```python
from build123d import *

# Parameters (mm, degrees)
SKETCH1_R               = 20.5
BOSS_EXTRUDE1_DEPTH     = 108
FILLET1_R               = 1
CUT_EXTRUDE1_REACH      = 130.166
CUT_EXTRUDE1_END_RADIUS = 18.5
CIRPATTERN1_COUNT       = 4
SKETCH7_R               = 0.75
BOSS_EXTRUDE2_DEPTH     = 0.5


# Read off the part's stored shape, not the designer's step: Shell1
with BuildPart() as part:
    # Sketch1 → Boss-Extrude1 (new body)
    with BuildSketch(Plane(origin=(0, 0, 0), x_dir=(1, 0, 0), z_dir=(0, 1, 0))):
        with Locations(Location((0, 0, 0), (0, 0, 270))):
            Circle(SKETCH1_R)
    extrude(amount=BOSS_EXTRUDE1_DEPTH)

    # Sketch3 → Revolve1 (revolve)
    with BuildSketch(Plane(origin=(0, 0, 0), x_dir=(0, 0, -1), z_dir=(1, 0, 0))):
        with BuildLine():
            Line((0, 116), (2.5, 116))
            Line((2.5, 116), (2.5, 114))
            ThreePointArc((2.5, 114), (5.663213274, 112.255038446), (8, 109.5))
            Line((8, 109.5), (8, 108))
            Line((8, 108), (0, 108))
            Line((0, 108), (0, 116))
        make_face()
    revolve(axis=Axis((0, 108, 0), (0, 1, 0)))

    # Fillet1
    fillet1_edges = [part.edges().sort_by_distance(p)[0] for p in [
        (0, 108, -20.5),
    ]]
    fillet(fillet1_edges, radius=FILLET1_R)

    # Shell1 outline → Shell1 (revolve, cut)
    with BuildSketch(Plane.XY):
        with BuildLine():
            Line((18.5, 0), (18.5, 106))
            Line((18.5, 106), (6, 106))
            Line((6, 106), (6, 108.933863711))
            ThreePointArc((6, 108.933863711), (3.622087212, 111.267143588), (0.5, 112.429570209))
            Line((0.5, 112.429570209), (0.5, 114))
            Line((0.5, 114), (0, 114))
            Line((0, 114), (0, 0))
            Line((0, 0), (18.5, 0))
        make_face()
    revolve(axis=Axis((0, 0, 0), (0, 1, 0)), mode=Mode.SUBTRACT)

    # Cut-Extrude1: up to this cylinder (the profile starts outside it)
    cut_extrude1_end = Plane(origin=(0, 80, 0), z_dir=(0, -1, 0)) * Cylinder(CUT_EXTRUDE1_END_RADIUS, 298.332, mode=Mode.PRIVATE)
    # Sketch4 → Cut-Extrude1 (cut, up to the surface)
    with BuildSketch(Plane(origin=(30, 0, 0), x_dir=(0, 0, -1), z_dir=(1, 0, 0)), mode=Mode.PRIVATE) as cut_extrude1_sk1:
        with BuildLine():
            Line((-7.5, 83), (7.5, 83))
            ThreePointArc((7.5, 83), (10.5, 80), (7.5, 77))
            Line((7.5, 77), (-7.5, 77))
            ThreePointArc((-7.5, 77), (-10.5, 80), (-7.5, 83))
        make_face()
    cut_extrude1_tool1 = extrude(cut_extrude1_sk1.sketch, amount=-CUT_EXTRUDE1_REACH, mode=Mode.PRIVATE) - cut_extrude1_end
    cut_extrude1 = cut_extrude1_tool1.solids().sort_by_distance((30, 80, 0))[0]
    add(cut_extrude1, mode=Mode.SUBTRACT)

    # CirPattern1: Cut-Extrude1 ×4 about axis
    cirpattern1_axis = Axis((0, 0, 0), (0, 1, 0))
    for i in range(1, CIRPATTERN1_COUNT):
        add(cut_extrude1.rotate(cirpattern1_axis, i * 360 / CIRPATTERN1_COUNT), mode=Mode.SUBTRACT)

    # Sketch7 → Boss-Extrude2 (add)
    with BuildSketch(Plane.XY.offset(15)):
        with BuildLine():
            Line((-1.5, 108), (1.5, 108))
            Line((1.5, 108), (1.5, 113))
            ThreePointArc((1.5, 113), (0, 114.5), (-1.5, 113))
            Line((-1.5, 113), (-1.5, 108))
        make_face()
        with Locations((0, 113)):
            Circle(SKETCH7_R, mode=Mode.SUBTRACT)
    boss_extrude2 = extrude(amount=BOSS_EXTRUDE2_DEPTH)

    # Mirror1: Boss-Extrude2 across plane
    add(boss_extrude2.mirror(Plane.XY))


solid = part.part
```
The model under review builds one solid part; all positions refer to its coordinate system, in mm. A direction names the side the tool comes from. Round coordinates to 2 decimals unless told otherwise and drop trailing zeros. Loops run counter-clockwise (first coordinate to the right, second up) from the corner with the lowest first, then second, coordinate; pieces in that order, holes last. Notation, with made-up numbers: (-16.5, 5) - (3.5, 5) arc R13 ccw to (3.5, 17) - close; hole circle Ø10 at (79, 56.5). An arc over 180 degrees is marked (long way). Use a Markdown table: item, result. Add a question column.
Q1. For probe 1 along Y at (x, z) = (0, 15.1); probe 2 along X at (y, z) = (113, 15.1); probe 3 along Z at (x, y) = (0, 54), list the stretches that pass through material, from the lowest coordinate up.
Q2. Insertion check: pin 1 Ø0.6 at (y, z) = (109.5, 15) entering from -X; pin 2 Ø1 at (y, z) = (78.5, -8) entering from -X; pin 3 Ø1.5 at (x, y) = (5.5, 41) entering from -Z; pin 4 Ø2.5 at (x, y) = (0, 113) entering from +Z. Each pin has a flat end and moves straight along its axis. Give the tip position at first contact, or say it passes through.
Q3. Machinability: for faces 5 (the face through (7.81, 108.74, 1.73)), 6 (the face through (0, 111, 15)), 7 (the face through (0, 77, 19)), 8 (the face through (0, 111, -15.5)), 9 (the face through (-17.2, 79.9, -10.5)), which of the approach directions +Z, -Z, +X, -X, +Y, -Y give a long, thin tool a straight path to every point of the face, cutting with its end or side? Answer none if there is none.
Q4. The part is to be moulded in two halves that separate along Z. For faces 1 (the face through (-6, 107, 0)), 2 (the face through (0, 83, -19)), 3 (the face through (-20.013, 52.751, -4.444)), 4 (the face through (0, 111, 15.5)), say which applies: pulls with the +Z half, pulls with the -Z half, needs draft (parallel to the pull), parting line crosses it, or undercut.
Q5. Add section A-A (y = 80). State the section outline as (x, z) points, plus the area to 3 significant figures.
Worked answers:
| question | item | result |
|---|---|---|
| 1 | probe 1 | 106 to 112.25, 113.75 to 114.5 |
| 1 | probe 2 | -1.5 to -0.75, 0.75 to 1.5 |
| 1 | probe 3 | -20.5 to -18.5, 18.5 to 20.5 |
| 2 | pin 1 | x = -1.5 |
| 2 | pin 2 | through |
| 2 | pin 3 | z = -19.94 |
| 2 | pin 4 | z = 15.5 |
| 3 | face 5 | +Y |
| 3 | face 6 | +X, -X, +Y |
| 3 | face 7 | +Z, -Z |
| 3 | face 8 | -Z, +X, -X, +Y |
| 3 | face 9 | +X, -X |
| 4 | face 1 | undercut |
| 4 | face 2 | needs draft |
| 4 | face 3 | parting line crosses it |
| 4 | face 4 | pulls with the +Z half |
| 5 | outline | (-17.61, -10.5) arc R20.5 ccw to (-10.5, -17.61) - (-10.5, -15.23) arc R18.5 cw to (-15.23, -10.5) - close; (-17.61, 10.5) - (-15.23, 10.5) arc R18.5 cw to (-10.5, 15.23) - (-10.5, 17.61) arc R20.5 ccw to start; (10.5, -17.61) arc R20.5 ccw to (17.61, -10.5) - (15.23, -10.5) arc R18.5 cw to (10.5, -15.23) - close; (10.5, 15.23) arc R18.5 cw to (15.23, 10.5) - (17.61, 10.5) arc R20.5 ccw to (10.5, 17.61) - close |
| 5 | area | 67.6 mm² |
